Build history of the part. All positions in model axes, mm. Face numbers are marked on the shaded views. A direction names the side the tool comes from. Give positions to 0.01 mm unless a question says otherwise; leave off trailing zeros. Write each loop counter-clockwise with the first axis right and the second up, starting at its lowest first coordinate (ties: lowest second). Pieces come first, ordered by that corner, then holes. Notation, with made-up numbers: (9.5, 3) -> (65.5, 3) arc R22 cw to (65.5, 35) -> close; hole circle Ø3 at (-36.75, 60). An arc over 180 degrees is marked (long way). One line per question, with ' | ' between items. Start each with the question number.
(1) Band-saw the part on B-B, the plane y = 35. Give the cut face in (x, z).
(2) Drill centre lines: probe 1 along Z at (x, y) = (1.8, 35); probe 2 along X at (y, z) = (19.5, 11). Where is each one in solid material? Low to high. Write a range as from..to.
(3) Band-saw the part on D-D, the plane y = 52.5. Give the cut face in (x, z), and give its area (3 significant figures).
(4) Tool access for the marked faces 1 and 2: list every direction of +Z, -Z, +X, -X, +Y, -Y with a clear straight run to the whole face (end or side of a thin tool).
(5) Band-saw the part on C-C, the plane z = 5.5. Give the cut face in (x, y), and give its area (3 significant figures).
(6) Pin check, flat tips, straight feed: P1, Ø6, axis at y = 14, z = 61, coming from the +X side; P2, Ø20, axis at x = 43, z = 34, coming from the +Y side. Stop position of each tip, or through.
(7) Band-saw the part on A-A, the plane z = 35. Give the cut face in (x, y).
from build123d import *

# Parameters (mm, degrees)
BOSS_EXTRU_1_DEPTH      = 70
ESQUISSE2_R             = 11
ENL_V_MAT_EXTRU_1_DEPTH = 70
CONG_8_R                = 1
CONG_9_R                = 1


with BuildPart() as part:
    # Esquisse1 → Boss.-Extru.1 (new body)
    with BuildSketch(Plane.XY):
        Polygon((0, 0), (70, 0), (70, 3), (3, 3), (3, 70), (0, 70), align=None)
    extrude(amount=BOSS_EXTRU_1_DEPTH)

    # Esquisse2 → Enlèv. mat.-Extru.1 (cut)
    with BuildSketch(Plane(origin=(3, 0, 0), x_dir=(0, 0, -1), z_dir=(1, 0, 0))):
        with Locations(Location((-35, 35, 0), (0, 0, 90))):  # turned: the seam where the file's is
            Circle(ESQUISSE2_R)
    extrude(amount=-ENL_V_MAT_EXTRU_1_DEPTH, mode=Mode.SUBTRACT)

    # Congé8
    cong_8_edges = [part.edges().sort_by_distance(p)[0] for p in [
        (0, 0, 35),
    ]]
    fillet(cong_8_edges, radius=CONG_8_R)

    # Congé9
    cong_9_edges = [part.edges().sort_by_distance(p)[0] for p in [
        (1.5, 70, 70),
        (1.5, 70, 0),
    ]]
    fillet(cong_9_edges, radius=CONG_9_R)


solid = part.part
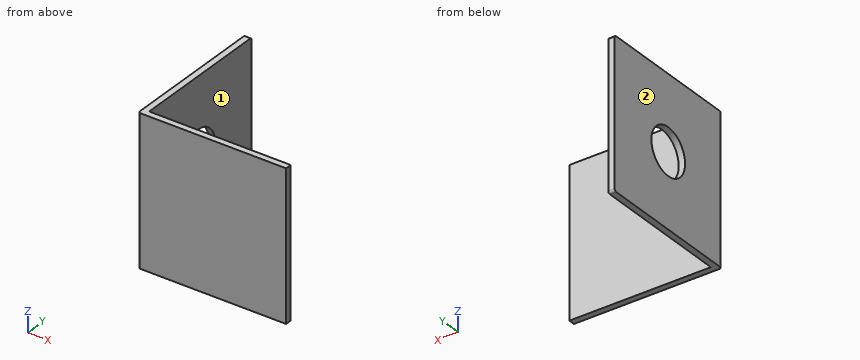
Results:
1) outline: (0, 0) -> (3, 0) -> (3, 24) -> (0, 24) -> close; (0, 46) -> (3, 46) -> (3, 70) -> (0, 70) -> close
2) probe 1: z = 0..24, 46..70 | probe 2: x = 0..3
3) outline: (0, 0) -> (3, 0) -> (3, 70) -> (0, 70) -> close | area: 210 mm²
4) face 1: +Z, -Z, +X, +Y | face 2: +Z, -Z, -X, +Y, -Y
5) outline: (0, 1) arc R1 ccw to (1, 0) -> (70, 0) -> (70, 3) -> (3, 3) -> (3, 70) -> (0, 70) -> close | area: 411 mm²
6) P1: stops at x = 3 | P2: stops at y = 3
7) outline: (0, 1) arc R1 ccw to (1, 0) -> (70, 0) -> (70, 3) -> (3, 3) -> (3, 24) -> (0, 24) -> close; (0, 46) -> (3, 46) -> (3, 70) -> (0, 70) -> close
